from build123d import *

# Parameters (mm, degrees)
F0_W     = 50.8
F0_H     = 50.8
F0_W_2   = 47.498
F0_H_2   = 47.498
F1_DEPTH = 1422.4
F2_R     = 1.651
F3_R     = 1.651


with BuildPart() as f1:
    # F0 (on Front) → F1 (new body)
    with BuildSketch(Plane.XZ):
        Rectangle(F0_W, F0_H)
        Rectangle(F0_W_2, F0_H_2, mode=Mode.SUBTRACT)
    extrude(amount=-F1_DEPTH)

    # F2
    f2_edges = [f1.edges().sort_by_distance(p)[0] for p in [
        (-23.749, 711.2, 23.749),
        (23.749, 711.2, 23.749),
        (-23.749, 711.2, -23.749),
        (23.749, 711.2, -23.749),
    ]]
    fillet(f2_edges, radius=F2_R)

    # F3
    f3_edges = [f1.edges().sort_by_distance(p)[0] for p in [
        (-25.4, 711.2, 25.4),
        (-25.4, 711.2, -25.4),
        (25.4, 711.2, 25.4),
        (25.4, 711.2, -25.4),
    ]]
    fillet(f3_edges, radius=F3_R)


solid = f1.part
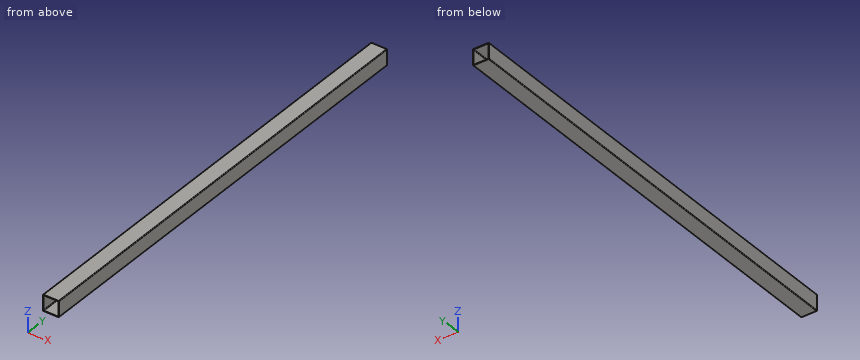
Model file for the job. Use its own axes, mm. Round coordinates to 2 decimals unless told otherwise and drop trailing zeros. Order: outer loops, then holes, each group sorted by start corner. A loop starts at its lowest first (then second) coordinate and runs counter-clockwise, first axis right, second up.
(1) Drill centre line: line 1 (X direction, y = 797, z = -18.5). Where is it in solid material? Low to high.
(2) Band-saw the part on B-B (z = -6). List the corners of the cut face in (x, y).
(3) Band-saw the part on C-C (y = 104). List the corners of the cut face in (x, z), then the cut area to 3 significant figures.
(4) Band-saw the part on A-A (x = 6). List the corners of the cut face in (y, z), then the cut area to 3 significant figures.
Verdict:
1. line 1: x = -25.4 to -23.75, 23.75 to 25.4
2. outline: (-25.4, 0) - (-23.75, 0) - (-23.75, 1422.4) - (-25.4, 1422.4) - close; (23.75, 0) - (25.4, 0) - (25.4, 1422.4) - (23.75, 1422.4) - close
3. outline: (-25.4, -23.75) arc R1.65 ccw to (-23.75, -25.4) - (23.75, -25.4) arc R1.65 ccw to (25.4, -23.75) - (25.4, 23.75) arc R1.65 ccw to (23.75, 25.4) - (-23.75, 25.4) arc R1.65 ccw to (-25.4, 23.75) - close; hole (-23.75, -22.1) arc R1.65 ccw to (-22.1, -23.75) - (22.1, -23.75) arc R1.65 ccw to (23.75, -22.1) - (23.75, 22.1) arc R1.65 ccw to (22.1, 23.75) - (-22.1, 23.75) arc R1.65 ccw to (-23.75, 22.1) - close
3. area: 325 mm2
4. outline: (0, -25.4) - (1422.4, -25.4) - (1422.4, -23.75) - (0, -23.75) - close; (0, 23.75) - (1422.4, 23.75) - (1422.4, 25.4) - (0, 25.4) - close
4. area: 4,700 mm2
